Could you check a few things on this model? Use its own coordinates, in mm. Face numbers are marked on the shaded views. A direction names the side the tool comes from. Give positions to 0.01 mm unless a question says otherwise; leave off trailing zeros. Write each loop counter-clockwise with the first axis right and the second up, starting at its lowest first coordinate (ties: lowest second). Pieces come first, ordered by that corner, then holes. Notation, with made-up numbers: (55.25, 20.25) - (62.25, 20.25) arc R20 cw to (62.25, 37.25) - close; hole circle Ø3 at (-13, 71). An arc over 180 degrees is marked (long way). Write item = value, one per line.
from build123d import *

# Parameters (mm, degrees)
SKETCH_1_W              = 7.25
SKETCH_1_H              = 3
EXTRUDE_1_REACH         = 30.357
EXTRUDE_1_END_RADIUS    = 7.25
SKETCH_2_W              = 1
SKETCH_2_H              = 7
SKETCH_3_R              = 4.25
EXTRUDE_2_DEPTH         = 5
HOLE_WIZARD_5_5_5_5_1_D = 5.5


with BuildPart() as part:
    # Эскиз1 → Повернуть1 (revolve)
    with BuildSketch(Plane.XZ, mode=Mode.PRIVATE) as revolve_1_sk:
        with Locations((3.625, 1.5)):
            Rectangle(SKETCH_1_W, SKETCH_1_H)
    revolve(revolve_1_sk.sketch.rotate(Axis((0, 0, 3), (0, 0, -1)), 180), axis=Axis((0, 0, 3), (0, 0, -1)))

    # Бобышка-Вытянуть1: up to this cylinder (the profile starts outside it)
    extrude_1_end = Plane(origin=(0, 0, 2.5), z_dir=(0, 0, -1)) * Cylinder(EXTRUDE_1_END_RADIUS, 76.214, mode=Mode.PRIVATE)
    # Эскиз2 → Бобышка-Вытянуть1 (add, up to the surface)
    with BuildSketch(Plane(origin=(20, 0, 0), x_dir=(0, 0, -1), z_dir=(1, 0, 0)), mode=Mode.PRIVATE) as extrude_1_sk1:
        with Locations((-2.5, 0)):
            Rectangle(SKETCH_2_W, SKETCH_2_H)
    extrude_1_tool1 = extrude(extrude_1_sk1.sketch, amount=-EXTRUDE_1_REACH, mode=Mode.PRIVATE) - extrude_1_end
    add(extrude_1_tool1.solids().sort_by_distance((20, 0, 2.5))[0])

    # Эскиз3 → Бобышка-Вытянуть2 (add)
    with BuildSketch(Plane(origin=(0, 0, 0), x_dir=(-1, 0, 0), z_dir=(0, 0, -1))):
        Circle(SKETCH_3_R)
    extrude(amount=EXTRUDE_2_DEPTH)

    # Диаметр отверстия Ø5.5 (5.5)1 (through all)
    with Locations(Plane.XY.offset(3)):
        with Locations((0, 0)):
            Hole(HOLE_WIZARD_5_5_5_5_1_D / 2)


solid = part.part
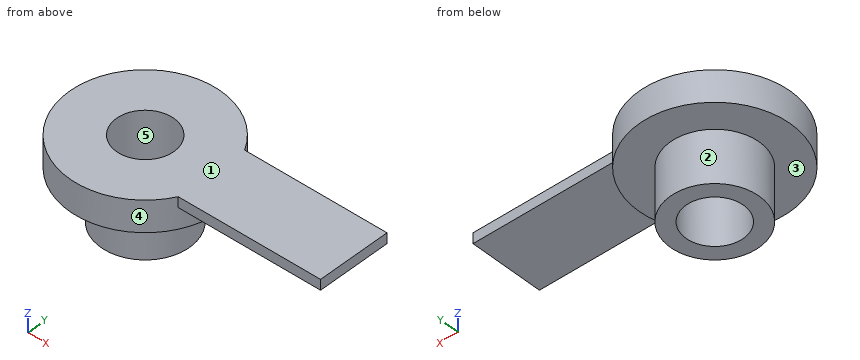
1. If we section it at C-C, the plane z = 1.5: Please give me the cut outline in (x, y).
Filled sheet:
outline = circle Ø14.5 at (0, 0); hole circle Ø5.5 at (0, 0)
2. Which directions (+Z, -Z, +X, -X, +Y, -Y) give clear straight access to the entire face, cutting with the end or side of a thin tool? Please do the marked faces 1 and 2.
Filled sheet:
face_1 = +Z, +X, -X, +Y, -Y
face_2 = -Z
3. I need wall thicknesses on line 1 (Y direction, x = 0, z = -3); line 2 (Z direction, x = 8.5, y = -2.5); line 3 (X direction, y = -1.75, z = -4.25). Which ranges of each line are inside material? Lowest first, please.
Filled sheet:
line_1 = -4.25 to -2.75, 2.75 to 4.25
line_2 = 2 to 3
line_3 = -3.87 to -2.12, 2.12 to 3.87
4. If we section it at A-A, the plane x = 0: Please give me the cut outline in (y, z), and give its area (3 significant figures).
Filled sheet:
outline = (-7.25, 0) - (-4.25, 0) - (-4.25, -5) - (-2.75, -5) - (-2.75, 3) - (-7.25, 3) - close; (2.75, -5) - (4.25, -5) - (4.25, 0) - (7.25, 0) - (7.25, 3) - (2.75, 3) - close
area = 42.0 mm2
5. Thinking about a two-plate mould opening in Y: for the marked faces 3, 4 and 5, which applies, pulls with the +Y half, pulls with the -Y half, needs draft (parallel to the pull), parting line crosses it, or undercut?
Filled sheet:
face_3 = needs draft
face_4 = parting line crosses it
face_5 = undercut
6. For pin 1 (2 mm diameter, centred on x = 16.5, y = -0.5, fed in from -Z); pin 2 (1.1 mm diameter, centred on x = 16, z = 2.5, fed in from +Y); pin 3 (3 mm diameter, centred on y = -1.5, z = -1, fed in from +X), each with a flat end and sliding along its axis, tell me the tip position at first contact or that it passes through.
Filled sheet:
pin_1 = 2
pin_2 = 3.5
pin_3 = 7.24
7. If we section it at B-B, the plane y = 0: Please give me the cut outline in (x, z).
Filled sheet:
outline = (-7.25, 0) - (-4.25, 0) - (-4.25, -5) - (-2.75, -5) - (-2.75, 3) - (-7.25, 3) - close; (2.75, -5) - (4.25, -5) - (4.25, 0) - (7.25, 0) - (7.25, 2) - (20, 2) - (20, 3) - (2.75, 3) - close
8. If we section it at D-D, the plane x = 11: Please give me the cut outline in (y, z), and give its area (3 significant figures).
Filled sheet:
outline = (-3.5, 2) - (3.5, 2) - (3.5, 3) - (-3.5, 3) - close
area = 7.00 mm2
